Could you check a few things on this drawing? It's one solid part, dimensions in mm from its lowest x, y, z. Round coordinates to 2 decimals unless told otherwise and drop trailing zeros. Order: outer loops, then holes, each group sorted by start corner. A loop starts at its lowest first (then second) coordinate and runs counter-clockwise, first axis right, second up. Notation, with made-up numbers: (8.5, 13.25) -> (52.5, 13.25) arc R20 ccw to (52.5, 41.25) -> close; hole circle Ø10 at (-40, 24). An arc over 180 degrees is marked (long way). Use a Markdown table: item, result. Add a question column.
(1) I want a section at B-B, the plane x = 61.5. Please give me the cut outline in (y, z), then the cut area to 3 significant figures.
(2) I want a section at C-C, the plane z = 4. Please give me the cut outline in (x, y).
(3) If I drill on probe 1 along Y at (x, z) = (57, 3.5); probe 2 along Z at (x, y) = (43.5, 29); probe 3 along X at (y, z) = (46.5, 5.75), over which ranges is the centre line in solid material (lowest first)?
(4) I want a section at D-D, the plane x = 20.5. Please give me the cut outline in (y, z).
(5) I'm going to push flat-ended pins straight in: P1, Ø4, axis at y = 46, z = 2.5, coming from the +X side; P2, Ø4, axis at x = 51, y = 19, coming from the -Z side; P3, Ø1.4, axis at y = 47.5, z = 4, coming from the -X side. Where does each tip first touch, or does it pass through?
(6) I want a section at A-A, the plane y = 45.5. Please give me the cut outline in (x, z), then the cut area to 3 significant figures.
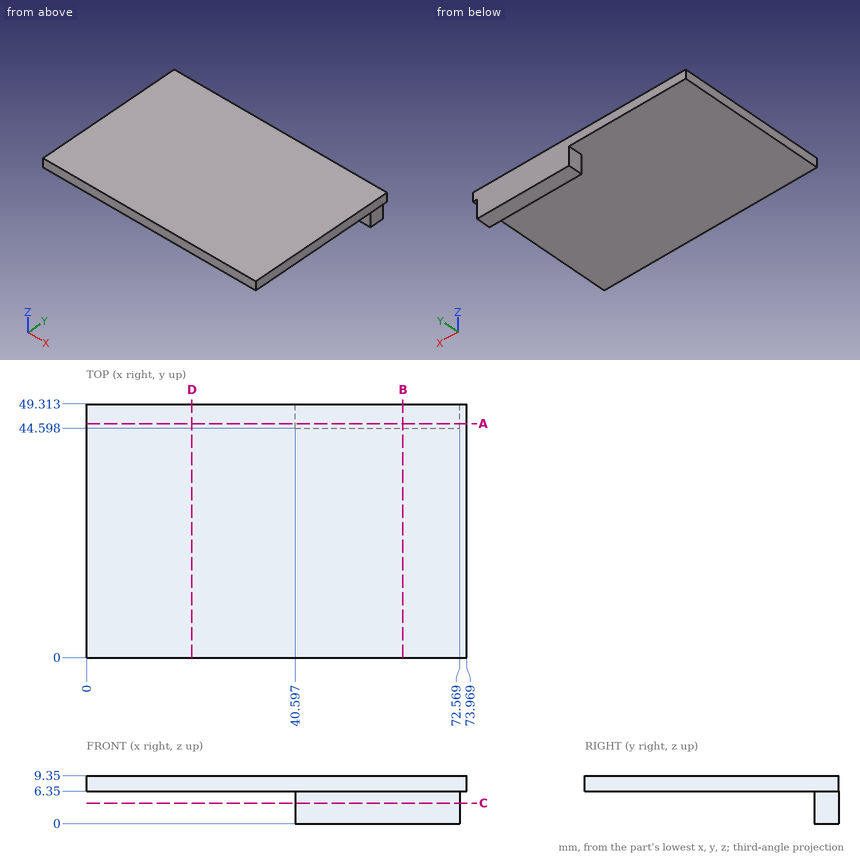
Taken from the geometry:
| question | item | result |
|---|---|---|
| 1 | outline | (0, 6.35) -> (44.6, 6.35) -> (44.6, 0) -> (49.31, 0) -> (49.31, 9.35) -> (0, 9.35) -> close |
| 1 | area | 178 mm2 |
| 2 | outline | (40.6, 44.6) -> (72.57, 44.6) -> (72.57, 49.31) -> (40.6, 49.31) -> close |
| 3 | probe 1 | y = 44.6 to 49.31 |
| 3 | probe 2 | z = 6.35 to 9.35 |
| 3 | probe 3 | x = 40.6 to 72.57 |
| 4 | outline | (0, 6.35) -> (49.31, 6.35) -> (49.31, 9.35) -> (0, 9.35) -> close |
| 5 | P1 | stops at x = 72.57 |
| 5 | P2 | stops at z = 6.35 |
| 5 | P3 | stops at x = 40.6 |
| 6 | outline | (0, 6.35) -> (40.6, 6.35) -> (40.6, 0) -> (72.57, 0) -> (72.57, 6.35) -> (73.97, 6.35) -> (73.97, 9.35) -> (0, 9.35) -> close |
| 6 | area | 425 mm2 |
